Model file for the job. Use its own axes, mm. Face numbers are marked on the shaded views. Round coordinates to 2 decimals unless told otherwise and drop trailing zeros. Loops run counter-clockwise (first coordinate to the right, second up) from the corner with the lowest first, then second, coordinate; pieces in that order, holes last. Notation, with made-up numbers: (38.25, 21.25) -> (81.25, 21.25) arc R25 ccw to (81.25, 34.25) -> close; hole circle Ø7 at (46, -12.75). An arc over 180 degrees is marked (long way). Use a Markdown table: item, result. Add a question column.
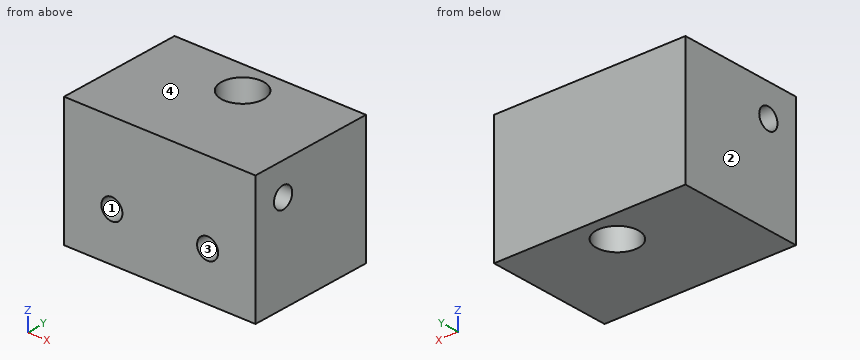
```python
from build123d import *

# Parameters (mm, degrees)
SKIZZE1_W                       = 30
SKIZZE1_H                       = 20
AUFSATZ_LINEAR_AUSTRAGEN1_DEPTH = 20
M6_GEWINDEBOHRUNG_D             = 3.3
M6_GEWINDEBOHRUNG_DEPTH         = 10.508579979
M6_GEWINDEBOHRUNG_TIP           = 0.991420021
DURCHGANGSLOCH_F_R_M61_D        = 6.6
M4_GEWINDEBOHRUNG1_D            = 3.3
M4_GEWINDEBOHRUNG1_DEPTH        = 14.008579979
M4_GEWINDEBOHRUNG1_TIP          = 0.991420021
M4_GEWINDEBOHRUNG2_D            = 3.3
M4_GEWINDEBOHRUNG2_DEPTH        = 15
M4_GEWINDEBOHRUNG2_TIP          = 0.991420021


with BuildPart() as part:
    # Skizze1 → Aufsatz-Linear austragen1 (new body)
    with BuildSketch(Plane.XY):
        with Locations((15, 10)):
            Rectangle(SKIZZE1_W, SKIZZE1_H)
    extrude(amount=AUFSATZ_LINEAR_AUSTRAGEN1_DEPTH)

    # M6 Gewindebohrung
    with Locations(Plane(origin=(0, 0, 0), x_dir=(-1, 0, 0), z_dir=(0, -1, 0))):
        with Locations((-22.5, -7.5), (-7.5, -7.5)):
            Hole(M6_GEWINDEBOHRUNG_D / 2, depth=M6_GEWINDEBOHRUNG_DEPTH)
            with Locations((0, 0, -(M6_GEWINDEBOHRUNG_DEPTH + M6_GEWINDEBOHRUNG_TIP / 2))):  # 118° drill point
                Cone(0, M6_GEWINDEBOHRUNG_D / 2, M6_GEWINDEBOHRUNG_TIP, mode=Mode.SUBTRACT)

    # Durchgangsloch für M61 (through all)
    with Locations(Plane.XY.offset(20)):
        with Locations((15, 15)):
            Hole(DURCHGANGSLOCH_F_R_M61_D / 2)

    # M4 Gewindebohrung1
    with Locations(Plane(origin=(30, 0, 0), x_dir=(0, 0, -1), z_dir=(1, 0, 0))):
        with Locations((-15, 5)):
            Hole(M4_GEWINDEBOHRUNG1_D / 2, depth=M4_GEWINDEBOHRUNG1_DEPTH)
            with Locations((0, 0, -(M4_GEWINDEBOHRUNG1_DEPTH + M4_GEWINDEBOHRUNG1_TIP / 2))):  # 118° drill point
                Cone(0, M4_GEWINDEBOHRUNG1_D / 2, M4_GEWINDEBOHRUNG1_TIP, mode=Mode.SUBTRACT)

    # M4 Gewindebohrung2
    with Locations(Plane.ZY):
        with Locations((15, 5)):
            Hole(M4_GEWINDEBOHRUNG2_D / 2, depth=M4_GEWINDEBOHRUNG2_DEPTH)
            with Locations((0, 0, -(M4_GEWINDEBOHRUNG2_DEPTH + M4_GEWINDEBOHRUNG2_TIP / 2))):  # 118° drill point
                Cone(0, M4_GEWINDEBOHRUNG2_D / 2, M4_GEWINDEBOHRUNG2_TIP, mode=Mode.SUBTRACT)


solid = part.part
```
1) Pull direction X, two halves, no side cores. Call the marked faces 1, 2, 3 and 4: +X half, -X half, draft (parallel to the pull), parting line (faces both ways), or undercut.
2) Cut at B-B on y = 15. Write the cut outline in (x, z).
3) Cut at A-A on y = 5. Write the cut outline in (x, z) (3 decimals), and give its area (3 significant figures).
4) Cut at C-C on z = 15. Write the cut outline in (x, y) (3 decimals).
5) Cut at D-D on x = 25.75. Write the cut outline in (y, z), and give its area (3 significant figures).
6) Wall check: probe 1 along X at (y, z) = (3.75, 7.5); probe 2 along Y at (x, z) = (15, 12.5); probe 3 along Z at (x, y) = (23.75, 5). Give the ranges that are in metal, low to high. Write a range as from..to.
Established:
| question | item | result |
|---|---|---|
| 1 | face 1 | undercut |
| 1 | face 2 | -X half |
| 1 | face 3 | undercut |
| 1 | face 4 | draft |
| 2 | outline | (0, 0) -> (11.7, 0) -> (11.7, 20) -> (0, 20) -> close; (18.3, 0) -> (30, 0) -> (30, 20) -> (18.3, 20) -> close |
| 3 | outline | (0, 0) -> (30, 0) -> (30, 13.35) -> (15.991, 13.35) -> (15.496, 14.175) -> (15, 13.35) -> (0, 13.35) -> close; (0, 16.65) -> (15, 16.65) -> (15.496, 15.825) -> (15.991, 16.65) -> (30, 16.65) -> (30, 20) -> (0, 20) -> close; hole circle Ø3.3 at (7.5, 7.5); hole circle Ø3.3 at (22.5, 7.5) |
| 3 | area | 485 mm^2 |
| 4 | outline | (0, 0) -> (30, 0) -> (30, 3.35) -> (15.991, 3.35) -> (15.496, 4.175) -> (15, 3.35) -> (0, 3.35) -> close; (0, 6.65) -> (15, 6.65) -> (15.496, 5.825) -> (15.991, 6.65) -> (30, 6.65) -> (30, 20) -> (0, 20) -> close; hole circle Ø6.6 at (15, 15) |
| 5 | outline | (0, 0) -> (20, 0) -> (20, 20) -> (0, 20) -> close; hole circle Ø3.3 at (5, 15) |
| 5 | area | 391 mm^2 |
| 6 | probe 1 | x = 0..5.85, 9.15..20.85, 24.15..30 |
| 6 | probe 2 | y = 0..11.7, 18.3..20 |
| 6 | probe 3 | z = 0..6.42, 8.58..13.35, 16.65..20 |
